Read the model definition and answer for the solid it produces. Units are mm, in the model's axes. A direction names the side the tool comes from. Coordinates: 2 decimals unless noted, no trailing zeros. Write each loop counter-clockwise with the first axis right and the second up, starting at its lowest first coordinate (ties: lowest second). Pieces come first, ordered by that corner, then holes. Notation, with made-up numbers: M 83.5,-37.5 L 95.5,-37.5 A28 ccw 95.5,-5.5 Z; hole C 16.25,80 d2. An arc over 180 degrees is marked long. Write item = value, one per line.
from build123d import *

# Parameters (mm, degrees)
SKETCH1_R           = 24.5
BOSS_EXTRUDE1_DEPTH = 57
SKETCH2_R           = 3
BOSS_EXTRUDE2_DEPTH = 21
FILLET1_R           = 2


with BuildPart() as part:
    # Sketch1 → Boss-Extrude1 (new body)
    with BuildSketch(Plane.XY):
        with Locations(Location((0, 0, 0), (0, 0, 180))):
            Circle(SKETCH1_R)
    extrude(amount=BOSS_EXTRUDE1_DEPTH)

    # Sketch2 → Boss-Extrude2 (add)
    with BuildSketch(Plane.XY.offset(57)):
        with Locations(Location((0, 0, 0), (0, 0, 180))):
            Circle(SKETCH2_R)
    extrude(amount=BOSS_EXTRUDE2_DEPTH)

    # Fillet1
    fillet1_edges = [part.edges().sort_by_distance(p)[0] for p in [
        (24.5, 0, 0),
        (24.5, 0, 57),
    ]]
    fillet(fillet1_edges, radius=FILLET1_R)


solid = part.part
Item 1: Consider line 1 along Z through (x, y) = (18, 0.5); line 2 along X through (y, z) = (-18.5, 43); line 3 along Y through (x, z) = (17, 52). Determine where each line is inside the solid, lowest interval first. Write a range as from..to.
Worked answers:
line_1 = 0..57
line_2 = -16.06..16.06
line_3 = -17.64..17.64
Item 2: Find section C-C (z = 72.5). Determine the outline of the cut face in (x, y).
Worked answers:
outline = C 0,0 d6
Item 3: Flat-ended cylindrical pins translate along their axes: pin 1 (2 mm diameter, centred on y = -10, z = 11, fed in from -X); pin 2 (8 mm diameter, centred on x = 15, z = 26.5, fed in from -Y); pin 3 (1 mm diameter, centred on y = 5, z = 53.5, fed in from -X). Find the tip coordinate at first contact, or state that the pin passes through.
Worked answers:
pin_1 = -22.79
pin_2 = -21.89
pin_3 = -24.08
Item 4: Find section A-A (y = 0). Determine the outline of the cut face in (x, z).
Worked answers:
outline = M -24.5,2 A2 ccw -22.5,0 L 22.5,0 A2 ccw 24.5,2 L 24.5,55 A2 ccw 22.5,57 L 3,57 L 3,78 L -3,78 L -3,57 L -22.5,57 A2 ccw -24.5,55 Z
Item 5: Which of the six approach directions +Z, -Z, +X, -X, +Y, -Y give full straight-line access (tool end or side, diameter ignored) to faces 1 (the face through (-13.17, -20.66, 28.13)), 2 (the face through (-2.86, -0.9, 67.35))?
Worked answers:
face_1 = +Z, -Z
face_2 = +Z
